```python
from build123d import *

# Parameters (mm, degrees)
CYLINDER156_R             = 2.2
CYLINDER156_DEPTH         = 50
FUSION076_PLACEMENT_ANGLE = 90
BOX068_W                  = 39
BOX068_H                  = 10
BOX068_DEPTH              = 8
CUT144_ROLL_ANGLE         = 180
CUT144_PLACEMENT_ANGLE    = 90


with BuildPart() as cylinder156:
    # Cylinder156 → Cylinder156 (new body)
    with BuildSketch(Plane(origin=(-24, 26, -8), x_dir=(0, 0, -1), z_dir=(1, 0, 0))):
        Circle(CYLINDER156_R)
    extrude(amount=CYLINDER156_DEPTH)


with BuildPart() as fusion076:
    # Cone018 → Cone018 (revolve)
    with BuildSketch(Plane(origin=(-24, 26, -8), x_dir=(0, 0, 1), z_dir=(0, -1, 0))):
        Polygon((0, 0), (2.2, 0), (4, 5), (0, 5), align=None)
    revolve(axis=Axis((-24, 26, -8), (-1, 0, 0)))

    # Fusion076: union Cylinder156
    add(cylinder156.part)


with BuildPart() as fusion076_1:
    # Fusion076 placement: moved
    add(fusion076.part.moved(Location((111.8, -1.7, 18.4))).rotate(Axis((111.8, -1.7, 18.4), (0, 1, 0)), FUSION076_PLACEMENT_ANGLE))


with BuildPart() as cut144:
    # Box068 → Box068 (new body)
    with BuildSketch(Plane(origin=(84.8, 19.5, 38.7), x_dir=(1, 0, 0), z_dir=(0, 0, 1))):
        with Locations((19.5, 5)):
            Rectangle(BOX068_W, BOX068_H)
    extrude(amount=BOX068_DEPTH)

    # Cut144: cut Fusion076
    add(fusion076_1.part, mode=Mode.SUBTRACT)


with BuildPart() as cut144_1:
    # Cut144 roll: moved
    add(cut144.part.rotate(Axis((0, 0, 0), (1, 0, 0)), CUT144_ROLL_ANGLE))


with BuildPart() as cut144_2:
    # Cut144 placement: moved
    add(cut144_1.part.moved(Location((96, 78.2, 103))).rotate(Axis((96, 78.2, 103), (0, 0, 1)), CUT144_PLACEMENT_ANGLE))


solid = cut144_2.part
```
Read the model definition and answer for the solid it produces. Units are mm, in the model's axes. Give positions to 0.01 mm unless a question says otherwise; leave off trailing zeros. Loops run counter-clockwise (first coordinate to the right, second up) from the corner with the lowest first, then second, coordinate; pieces in that order, holes last.
Item 1: The part is cut by section A-A (x = 120.3). Write down the section's boundary in (y, z).
Item 2: The part is cut by section D-D (z = 58.25). Write down the section's boundary in (x, y).
Item 3: The part is cut by section C-C (z = 63.25). Write down the section's boundary in (x, y).
Item 4: The mould has two halves that part along Y. Classify faces 1 (the flat face through (120, 202, 60)), 2 (the flat face through (121, 178, 56.3)), 3 (the conical face through (122.08, 180.05, 59.38)), 4 (the cylindrical face through (118.961, 183.746, 62.424)): released by +Y, released by -Y, zero draft, split by the parting line, or undercut.
Item 5: Find the intervals of material crossed by line 1 along X through (y, z) = (182, 61.6); line 2 along Y through (x, z) = (118.5, 57); line 3 along Y through (x, z) = (121, 60.25), in increasing order.
Item 6: The part is cut by section B-B (y = 182). Write down the section's boundary in (x, z), and give its area (3 significant figures).
Taken from the geometry:
1. outline: (163, 56.3) - (178.25, 56.3) - (179.8, 60.6) - (179.8, 64.3) - (163, 64.3) - close; (184.2, 60.6) - (185.75, 56.3) - (202, 56.3) - (202, 64.3) - (184.2, 64.3) - close
2. outline: (115.5, 163) - (125.5, 163) - (125.5, 202) - (115.5, 202) - close; hole circle Ø6.09 at (120.3, 182)
3. outline: (115.5, 163) - (125.5, 163) - (125.5, 202) - (115.5, 202) - close; hole circle Ø4.4 at (120.3, 182)
4. face 1: released by +Y
4. face 2: zero draft
4. face 3: undercut
4. face 4: undercut
5. line 1: x = 115.5 to 118.1, 122.5 to 125.5
5. line 2: y = 163 to 179, 185 to 202
5. line 3: y = 163 to 179.78, 184.22 to 202
6. outline: (115.5, 56.3) - (116.55, 56.3) - (118.1, 60.6) - (118.1, 64.3) - (115.5, 64.3) - close; (122.5, 60.6) - (124.05, 56.3) - (125.5, 56.3) - (125.5, 64.3) - (122.5, 64.3) - close
6. area: 38.1 mm2
